The figure shows three views and two pictorial views of one solid part (mm, origin at its lowest corner). Answer the questions. Give positions to 0.01 mm unless a question says otherwise; leave off trailing zeros. Loops run counter-clockwise (first coordinate to the right, second up) from the corner with the lowest first, then second, coordinate; pieces in that order, holes last. Notation, with made-up numbers: (-2, 9) - (56, 9) arc R10 ccw to (56, 18) - close; hole circle Ø3 at (-1, 75.5). An arc over 180 degrees is marked (long way). One line per question, with ' | ' between items.
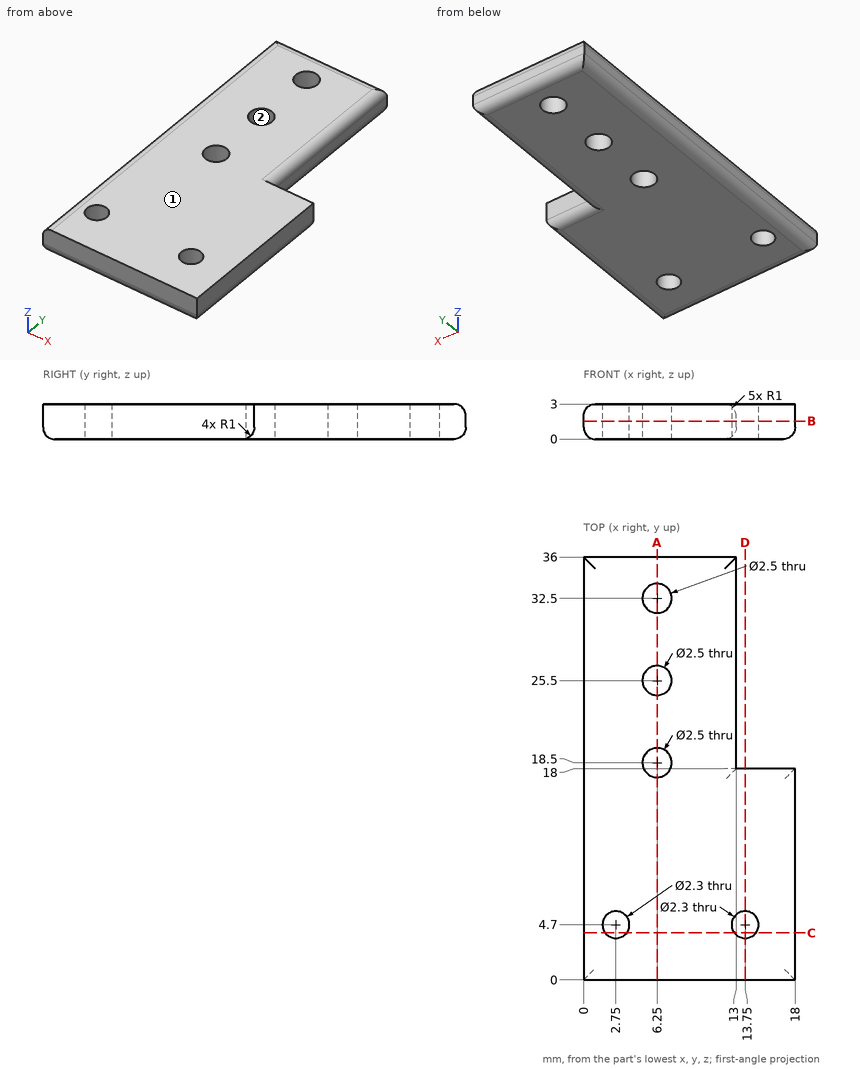
1. Find section A-A on x = 6.25. Write down the section's boundary in (y, z).
Evaluation:
outline: (0, 1) arc R1 ccw to (1, 0) - (17.25, 0) - (17.25, 3) - (0, 3) - close; (19.75, 0) - (24.25, 0) - (24.25, 3) - (19.75, 3) - close; (26.75, 0) - (31.25, 0) - (31.25, 3) - (26.75, 3) - close; (33.75, 0) - (35, 0) arc R1 ccw to (36, 1) - (36, 2) arc R1 ccw to (35, 3) - (33.75, 3) - close
2. Consider L1, parallel to Y at x = 6.25, z = 1.3; L2, parallel to Y at x = 13.75, z = 1.75; L3, parallel to Y at x = 6.5, z = 2.4. Determine where each line is inside the solid, lowest interval first.
Evaluation:
L1: 0 to 17.25, 19.75 to 24.25, 26.75 to 31.25, 33.75 to 36 | L2: 0 to 3.55, 5.85 to 18 | L3: 0 to 17.28, 19.72 to 24.28, 26.72 to 31.28, 33.72 to 35.92
3. Find section B-B on z = 1.55. Write down the section's boundary in (x, y), then the cut area to 3 significant figures.
Evaluation:
outline: (0, 0) - (18, 0) - (18, 18) - (13, 18) - (13, 36) - (0, 36) - close; hole circle Ø2.3 at (2.75, 4.7); hole circle Ø2.5 at (6.25, 18.5); hole circle Ø2.5 at (6.25, 25.5); hole circle Ø2.5 at (6.25, 32.5); hole circle Ø2.3 at (13.75, 4.7) | area: 535 mm2
4. A flat-ended cylindrical pin translates along its axis: pin 1 (1.6 mm diameter, centred on x = 14.5, z = 1.5, fed in from +Y). Find the tip coordinate at first contact, or state that the pin passes through.
Evaluation:
pin 1: y = 18
5. Find section D-D on x = 13.75. Write down the section's boundary in (y, z).
Evaluation:
outline: (0, 1) arc R1 ccw to (1, 0) - (3.55, 0) - (3.55, 3) - (0, 3) - close; (5.85, 0) - (17, 0) arc R1 ccw to (18, 1) - (18, 3) - (5.85, 3) - close
6. Find section C-C on y = 4. Write down the section's boundary in (x, z), then the cut area to 3 significant figures.
Evaluation:
outline: (0, 1) arc R1 ccw to (1, 0) - (1.84, 0) - (1.84, 3) - (1, 3) arc R1 ccw to (0, 2) - close; (3.66, 0) - (12.84, 0) - (12.84, 3) - (3.66, 3) - close; (14.66, 0) - (17, 0) arc R1 ccw to (18, 1) - (18, 3) - (14.66, 3) - close | area: 42.4 mm2
7. Determine the mould class of the marked faces 1 and 2 for opening direction Y: +Y half, -Y half, draft (parallel to the pull), parting line (faces both ways), or undercut.
Evaluation:
face 1: draft | face 2: undercut
